The listing builds one solid part. Answer for the finished solid, in the listing's coordinates (mm). Give positions to 0.01 mm unless a question says otherwise; leave off trailing zeros. Write each loop counter-clockwise with the first axis right and the second up, starting at its lowest first coordinate (ties: lowest second). Pieces come first, ordered by that corner, then holes. Notation, with made-up numbers: (69.25, 68) - (100.25, 68) arc R24 cw to (100.25, 94) - close; hole circle Ø11 at (-4.5, 60.25). An arc over 180 degrees is marked (long way). Write each question's results on one line, items separated by ' | '. Start each with the question number.
Q1. Section A-A (z = 49) is taken. Determine the outline of the cut face in (x, y).
Q2. Section C-C (x = 78) is taken. Determine the outline of the cut face in (y, z).
Q3. For a pull along Z with two mould halves and no side action, classify faces 1 (the face through (61, 0, 35)), 2 (the face through (138.673, 1.014, 46.858)), 3 (the face through (97.38, 0.99, 20.97)) as pulls with the +Z half, pulls with the -Z half, needs draft (parallel to the pull), parting line crosses it, or undercut.
Q4. Section D-D (z = 15) is taken. Determine the outline of the cut face in (x, y).
Q5. Section B-B (y = 1.25) is taken. Determine the outline of the cut face in (x, z).
Q6. Find the intervals of material crossed by probe 1 along Z at (x, y) = (137, 0.8); probe 2 along Z at (x, y) = (137.5, 0.3); probe 3 along X at (y, z) = (0.95, 51), in increasing order.
```python
from build123d import *

# Parameters (mm, degrees)
BOSS_EXTRUDE1_DEPTH = 2
SKETCH2_R           = 5
CUT_EXTRUDE1_DEPTH  = 165.132919655


with BuildPart() as part:
    # Sketch1 → Boss-Extrude1 (new body)
    with BuildSketch(Plane(origin=(0, 0, 0), x_dir=(1, 0, 0), z_dir=(0, 1, 0))):
        Polygon((0, 0), (42.592528424, 0), (153.715208146, -42.529795372), (153.715208146, -57.508695855), (0, -57.508695855), align=None)
    extrude(amount=BOSS_EXTRUDE1_DEPTH)

    # Sketch2 → Cut-Extrude1 (cut, through all)
    with BuildSketch(Plane(origin=(0, 2, 0), x_dir=(1, 0, 0), z_dir=(0, 1, 0))):
        with Locations(Location((133.715208146, -47.508695855, 0), (0, 0, 270))):
            Circle(SKETCH2_R)
    extrude(amount=-CUT_EXTRUDE1_DEPTH, mode=Mode.SUBTRACT)


solid = part.part
```
Answers below:
1) outline: (0, 0) - (128.94, 0) - (128.94, 2) - (0, 2) - close; (138.49, 0) - (153.72, 0) - (153.72, 2) - (138.49, 2) - close
2) outline: (0, 13.55) - (2, 13.55) - (2, 57.51) - (0, 57.51) - close
3) face 1: needs draft | face 2: undercut | face 3: pulls with the -Z half
4) outline: (0, 0) - (81.78, 0) - (81.78, 2) - (0, 2) - close
5) outline: (0, 0) - (42.59, 0) - (153.72, 42.53) - (153.72, 57.51) - (0, 57.51) - close; hole circle Ø10 at (133.72, 47.51)
6) probe 1: z = 36.13 to 43.74, 51.28 to 57.51 | probe 2: z = 36.32 to 44.24, 50.78 to 57.51 | probe 3: x = 0 to 130.14, 137.29 to 153.72
